```python
from build123d import *

# Parameters (mm, degrees)
SKETCH_W        = 50
SKETCH_H        = 30
PAD_DEPTH       = 5
SKETCH001_R     = 2.625
POCKET_DEPTH    = 5
SKETCH002_W     = 30
SKETCH002_H     = 30
PAD001_DEPTH    = 30
SKETCH003_W     = 20
SKETCH003_H     = 20
POCKET001_DEPTH = 30


with BuildPart() as part:
    # Sketch → Pad (new body)
    with BuildSketch(Plane.XZ):
        Rectangle(SKETCH_W, SKETCH_H)
    extrude(amount=PAD_DEPTH)

    # Sketch001 (on Face6 of Pad) → Pocket (cut)
    with BuildSketch(Plane.XZ.offset(5)):
        with Locations((-20, 10)):
            Circle(SKETCH001_R)
        with Locations((20, 10)):
            Circle(SKETCH001_R)
        with Locations((20, -10)):
            Circle(SKETCH001_R)
        with Locations((-20, -10)):
            Circle(SKETCH001_R)
    extrude(amount=-POCKET_DEPTH, mode=Mode.SUBTRACT)

    # Sketch002 (on Face5 of Pocket) → Pad001 (join)
    with BuildSketch(Plane.XZ.offset(5)):
        Rectangle(SKETCH002_W, SKETCH002_H)
    extrude(amount=PAD001_DEPTH)

    # Sketch003 (on Face9 of Pad001) → Pocket001 (cut)
    with BuildSketch(Plane(origin=(0, 0, 15), x_dir=(-1, 0, 0), z_dir=(0, 0, 1))):
        with Locations((0, 20)):
            Rectangle(SKETCH003_W, SKETCH003_H)
    extrude(amount=-POCKET001_DEPTH, mode=Mode.SUBTRACT)


solid = part.part
```
For this review, take the finished solid that the model builds, in its own axes (mm). A direction names the side the tool comes from. Coordinates: 2 decimals unless noted, no trailing zeros. Order: outer loops, then holes, each group sorted by start corner. A loop starts at its lowest first (then second) coordinate and runs counter-clockwise, first axis right, second up. Notation, with made-up numbers: (60.25, 58) -> (76.25, 58) arc R19 cw to (76.25, 72) -> close; hole circle Ø9 at (12.25, -17.5). An arc over 180 degrees is marked (long way). Use CSV: the item, a comma, the result in double quotes. Start each with the question number.
Item 1: Wall thickness on probe 1 along Z at (x, y) = (20, -2.8) (3 decimals); probe 2 along X at (y, z) = (-21, -6.75); probe 3 along Y at (x, z) = (1.5, -6.75): over which ranges is each line inside the solid? List them lowest first.
Item 2: We need section B-B, the plane x = 6. Give the boundary of the cut face in (y, z).
Item 3: We need section D-D, the plane x = 20. Give the boundary of the cut face in (y, z) (3 decimals), then the cut area to 3 significant figures.
Item 4: We need section A-A, the plane z = 10. Give the boundary of the cut face in (x, y) (3 decimals).
Item 5: For faces 1 (the face through (0, -30, 0)), 2 (the face through (17.92, -2.54, 8.4)), 3 (the face through (0, -35, 0)), 4 (the face through (-15, -20, 0)), 5 (the face through (15, -20, 0)), list the 3-axis set-ups (+Z, -Z, +X, -X, +Y, -Y) from which the entire face can be reached by the end or side of a thin tool; tool diameter is ignored.
Item 6: Draft analysis for pull direction Y (two halves, no side actions). For faces 6 (the face through (-10, -20, 0)), 7 (the face through (-20, -5, 0)), 8 (the face through (0, -10, 0)), 9 (the face through (-21.935, -2.535, -8.226)), state which applies: pulls with the +Y half, pulls with the -Y half, needs draft (parallel to the pull), parting line crosses it, or undercut.
Item 7: We need section C-C, the plane y = -18. Give the boundary of the cut face in (x, z), then the cut area to 3 significant figures.
Item 8: Insertion check: pin 1 (4 mm diameter, centred on x = 20, z = 10, fed in from +Y); pin 2 (6 mm diameter, centred on y = -23, z = 5, fed in from -X); pin 3 (10 mm diameter, centred on x = -1.5, z = -2, fed in from +Y); pin 4 (6 mm diameter, centred on y = -22, z = -5.5, fed in from +X). Each pin has a flat end and moves straight along its axis. Give the tip position at first contact, or say it passes through.
Derived:
1,probe 1,"z = -15 to -12.625, -7.375 to 7.375, 12.625 to 15"
1,probe 2,"x = -15 to -10, 10 to 15"
1,probe 3,"y = -35 to -30, -10 to 0"
2,outline,"(-35, -15) -> (-30, -15) -> (-30, 15) -> (-35, 15) -> close; (-10, -15) -> (0, -15) -> (0, 15) -> (-10, 15) -> close"
3,outline,"(-5, -15) -> (0, -15) -> (0, -12.625) -> (-5, -12.625) -> close; (-5, -7.375) -> (0, -7.375) -> (0, 7.375) -> (-5, 7.375) -> close; (-5, 12.625) -> (0, 12.625) -> (0, 15) -> (-5, 15) -> close"
3,area,"97.5 mm^2"
4,outline,"(-25, -5) -> (-22.625, -5) -> (-22.625, 0) -> (-25, 0) -> close; (-17.375, -5) -> (-15, -5) -> (-15, -35) -> (15, -35) -> (15, -5) -> (17.375, -5) -> (17.375, 0) -> (-17.375, 0) -> close; (22.625, -5) -> (25, -5) -> (25, 0) -> (22.625, 0) -> close; hole (-10, -30) -> (10, -30) -> (10, -10) -> (-10, -10) -> close"
5,face 1,"+Z, -Z"
5,face 2,"+Y, -Y"
5,face 3,"+Z, -Z, +X, -X, -Y"
5,face 4,"+Z, -Z, -X, -Y"
5,face 5,"+Z, -Z, +X, -Y"
6,face 6,"undercut"
6,face 7,"pulls with the -Y half"
6,face 8,"undercut"
6,face 9,"needs draft"
7,outline,"(-15, -15) -> (-10, -15) -> (-10, 15) -> (-15, 15) -> close; (10, -15) -> (15, -15) -> (15, 15) -> (10, 15) -> close"
7,area,"300 mm^2"
8,pin 1,"passes through"
8,pin 2,"stops at x = -15"
8,pin 3,"stops at y = 0"
8,pin 4,"stops at x = 15"
